For this review, take the finished solid that the model builds, in its own axes (mm). Face numbers are marked on the shaded views. A direction names the side the tool comes from. Give positions to 0.01 mm unless a question says otherwise; leave off trailing zeros. Write each loop counter-clockwise with the first axis right and the second up, starting at its lowest first coordinate (ties: lowest second). Pieces come first, ordered by that corner, then holes.
1) Machinability: for the marked faces 1 and 2, which of the approach directions +Z, -Z, +X, -X, +Y, -Y give a long, thin tool a straight path to every point of the face, cutting with its end or side? Answer none if there is none.
2) We need section A-A on x = 0. Give the boundary of the cut face in (y, z), and give its area (3 significant figures).
3) We need section D-D on y = -43. Give the boundary of the cut face in (x, z), and give its area (3 significant figures).
4) Wall thickness on line 1 along Z through (x, y) = (0.5, -37.5); line 2 along Y through (x, z) = (-0.5, -60); line 3 along Y through (x, z) = (-4, -82): over which ranges is each line inside the solid? List them lowest first.
5) For P1, Ø4, axis at y = -21.5, z = 25, coming from the -X side; P2, Ø1, axis at x = -20.5, y = -35.5, coming from the +Z side; P3, Ø5, axis at x = 2.5, z = -69.5, coming from the -Y side, all flat-tipped, find the tip position at first contact; note any pin that passes through.
6) We need section B-B on y = 0. Give the boundary of the cut face in (x, z), and give its area (3 significant figures).
7) We need section C-C on z = -46.5. Give the boundary of the cut face in (x, y), and give its area (3 significant figures).
from build123d import *

# Parameters (mm, degrees)
F0_R     = 42.5
F1_DEPTH = 50
F2_R     = 20
F3_DEPTH = 100
F4_W     = 10
F4_H     = 10
F5_DEPTH = 50


with BuildPart() as f1:
    # F0 (on Front) → F1 (new body, symmetric)
    with BuildSketch(Plane.XZ):
        Circle(F0_R)
    extrude(amount=F1_DEPTH, both=True)

    # F2 (on Top) → F3 (join)
    with BuildSketch(Plane.XY):
        Circle(F2_R)
    extrude(amount=-F3_DEPTH)

    # F4 (on face) → F5 (cut)
    with BuildSketch(Plane(origin=(0, 0, -100), x_dir=(1, 0, 0), z_dir=(0, 0, -1))):
        Rectangle(F4_W, F4_H)
    extrude(amount=-F5_DEPTH, mode=Mode.SUBTRACT)


solid = f1.part
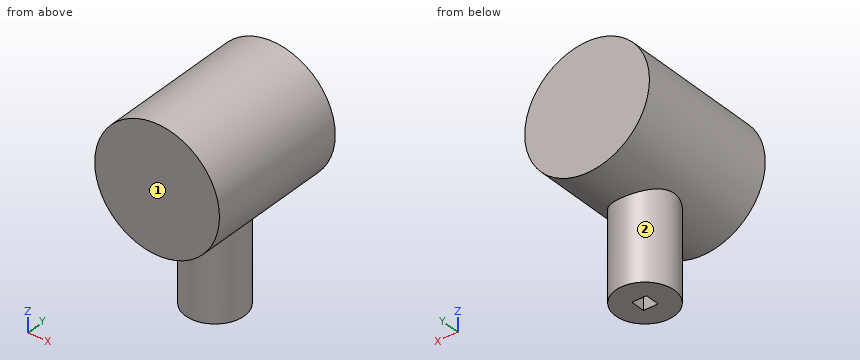
Results list:
1. face 1: +Z, -Z, +X, -X, -Y
1. face 2: -Z
2. outline: (-50, -42.5) - (-20, -42.5) - (-20, -100) - (-5, -100) - (-5, -50) - (5, -50) - (5, -100) - (20, -100) - (20, -42.5) - (50, -42.5) - (50, 42.5) - (-50, 42.5) - close
2. area: 10,300 mm2
3. outline: circle Ø85 at (0, 0)
3. area: 5,670 mm2
4. line 1: z = -42.5 to 42.5
4. line 2: y = -19.99 to -5, 5 to 19.99
4. line 3: y = -19.6 to -5, 5 to 19.6
5. P1: stops at x = -35.74
5. P2: stops at z = 37.5
5. P3: stops at y = -20
6. outline: (-20, -100) - (-5, -100) - (-5, -50) - (5, -50) - (5, -100) - (20, -100) - (20, -37.5) arc R42.5 ccw (long way) to (-20, -37.5) - close
6. area: 7,540 mm2
7. outline: circle Ø40 at (0, 0)
7. area: 1,260 mm2
